Verification items for this drawing (mm, ordinates from the low corner). Coordinates: 2 decimals unless noted, no trailing zeros. Order: outer loops, then holes, each group sorted by start corner. A loop starts at its lowest first (then second) coordinate and runs counter-clockwise, first axis right, second up. Notation, with made-up numbers: M 21,33.5 L 37,33.5 A23 cw 37,49.5 Z; hole C -6.5,3 d7. An arc over 180 degrees is marked long. Answer as a JSON object with one key per item and string values. Group by question number.
(1) Mould release check, pull along X, two halves, no side actions. Record for the marked faces 1, 2 and 3: released by +X, released by -X, zero draft, split by the parting line, or undercut.
(2) Cross-section at A-A (z = 52). Enter the section's corners in (x, y).
(3) Cross-section at D-D (y = 56.5). Enter the section's corners in (x, z), plus the area to 3 significant figures.
(4) Gauge pin test, flat ends, axial feed: pin 1 Ø11 at (x, y) = (35, 52.5) entering from -Z; pin 2 Ø5.5 at (x, z) = (86.5, 44) entering from +Y; pin 3 Ø5 at (x, z) = (21, 21.5) entering from +Y. Record the tip position at first contact, or that the pin passes through.
(5) Material ranges on line 1 (Y direction, x = 54, z = 57); line 2 (Y direction, x = 30.5, z = 29.5); line 3 (Z direction, x = 24.5, y = 51.5), recorded low to high.
(6) Cross-section at B-B (y = 28). Enter the section's corners in (x, z), plus the area to 3 significant figures.
(7) Cross-section at C-C (x = 20.5). Enter the section's corners in (y, z), plus the area to 3 significant figures.
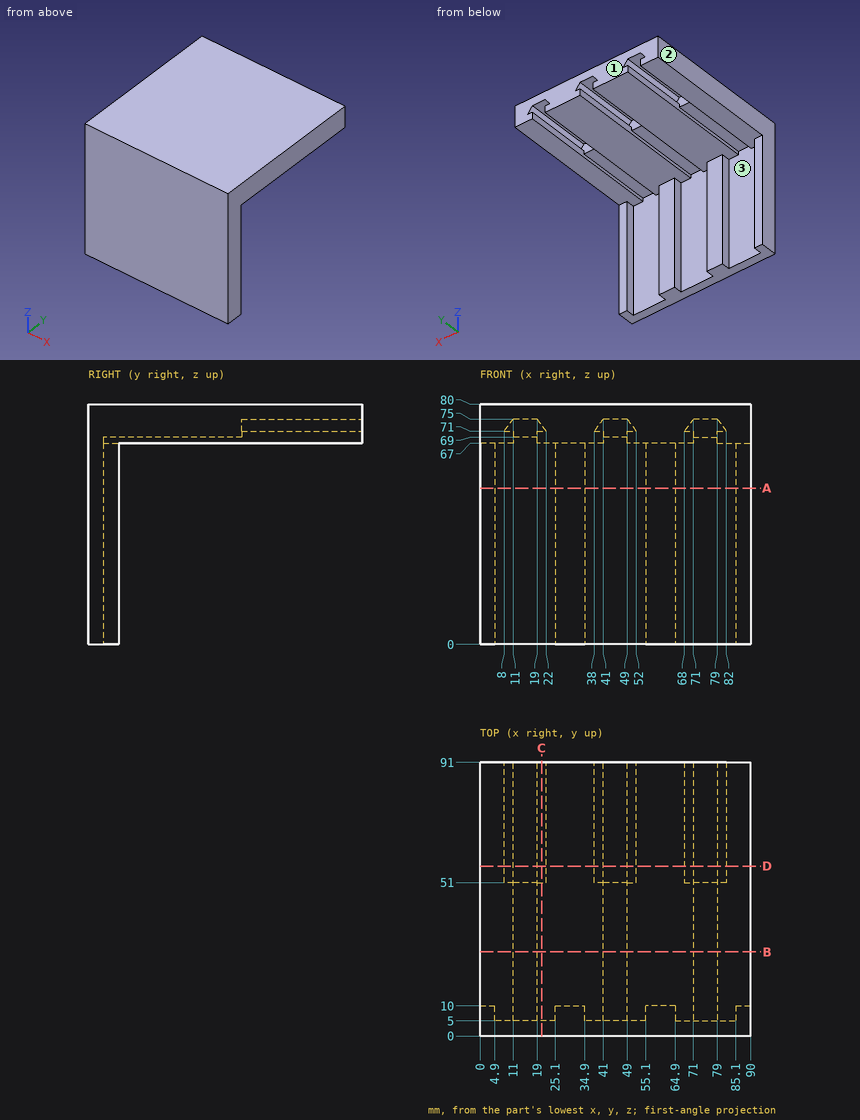
Taken from the geometry:
{
 "1": {"face 1": "zero draft", "face 2": "released by -X", "face 3": "undercut"},
 "2": {"outline": "M 0,0 L 90,0 L 90,10 L 85.1,10 L 85.1,5 L 64.9,5 L 64.9,10 L 55.1,10 L 55.1,5 L 34.9,5 L 34.9,10 L 25.1,10 L 25.1,5 L 4.9,5 L 4.9,10 L 0,10 Z"},
 "3": {"outline": "M 0,67 L 11,67 L 11,71 L 8,71 L 11,75 L 19,75 L 22,71 L 19,71 L 19,67 L 41,67 L 41,71 L 38,71 L 41,75 L 49,75 L 52,71 L 49,71 L 49,67 L 71,67 L 71,71 L 68,71 L 71,75 L 79,75 L 82,71 L 79,71 L 79,67 L 90,67 L 90,80 L 0,80 Z", "area": "942 mm²"},
 "4": {"pin 1": "stops at z = 67", "pin 2": "stops at y = 10", "pin 3": "stops at y = 5"},
 "5": {"line 1": "y = 0 to 5", "line 2": "y = 0 to 10", "line 3": "z = 67 to 80"},
 "6": {"outline": "M 0,67 L 11,67 L 11,69 L 19,69 L 19,67 L 41,67 L 41,69 L 49,69 L 49,67 L 71,67 L 71,69 L 79,69 L 79,67 L 90,67 L 90,80 L 0,80 Z", "area": "1,120 mm²"},
 "7": {"outline": "M 0,0 L 5,0 L 5,67 L 91,67 L 91,71 L 51,71 L 51,73 L 91,73 L 91,80 L 0,80 Z", "area": "1,440 mm²"}
}
